Design review of the part built by this model. Coordinates are the model's own, in mm. Face numbers are marked on the shaded views. A direction names the side the tool comes from. Coordinates: 2 decimals unless noted, no trailing zeros. Write each loop counter-clockwise with the first axis right and the second up, starting at its lowest first coordinate (ties: lowest second). Pieces come first, ordered by that corner, then holes. Notation, with made-up numbers: M 41,36.5 L 89,36.5 A13 cw 89,53.5 Z; hole C 9,15.5 d10. An arc over 180 degrees is marked long. Write each question's results on one line, items separated by ' | '. Start each with the question number.
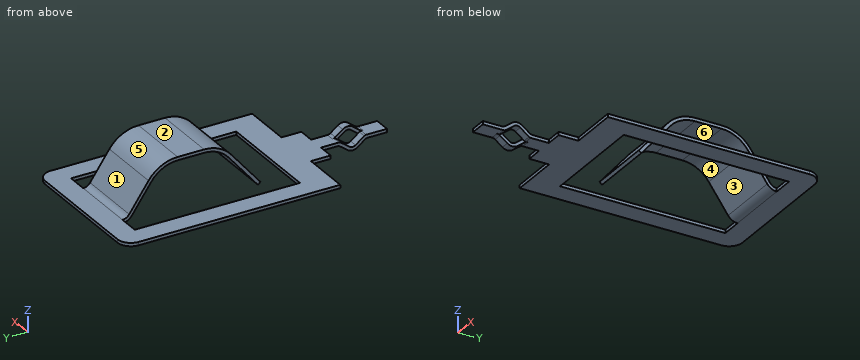
```python
from build123d import *

# Parameters (mm, degrees)
SKETCH1_W           = 6.5
SKETCH1_H           = 10
BOSS_EXTRUDE1_DEPTH = 0.2
BOSS_EXTRUDE2_DEPTH = 2
BOSS_EXTRUDE3_DEPTH = 0.5
FILLET1_R           = 0.8
BOSS_EXTRUDE7_DEPTH = 0.5


with BuildPart() as part:
    # Sketch1 → Boss-Extrude1 (new body)
    with BuildSketch(Plane.XY):
        Polygon((-4.5, 0), (4.5, 0), (4.5, -13), (1.5, -13), (1.5, -14.2), (-1.5, -14.2), (-1.5, -13), (-4.5, -13), align=None)
        with Locations((0, -6.3)):
            Rectangle(SKETCH1_W, SKETCH1_H, mode=Mode.SUBTRACT)
    extrude(amount=BOSS_EXTRUDE1_DEPTH)

    # Sketch2 → Boss-Extrude2 (add, symmetric)
    with BuildSketch(Plane.ZY):
        with BuildLine():
            Line((2.8, -4.64068371), (2.8, -6.24068371))
            ThreePointArc((2.8, -6.24068371), (2.617192211, -7.065276361), (2.103024175, -7.73535319))
            Line((2.103024175, -7.73535319), (0, -9.5))
            Line((0, -9.5), (0.128557522, -9.653208889))
            Line((0.128557522, -9.653208889), (2.231581697, -7.888562079))
            ThreePointArc((2.231581697, -7.888562079), (2.798453768, -7.149800013), (3, -6.24068371))
            Line((3, -6.24068371), (3, -4.64068371))
            ThreePointArc((3, -4.64068371), (2.756943079, -3.647392057), (2.082697913, -2.878562796))
            Line((2.082697913, -2.878562796), (0.413211782, -1.709576022))
            ThreePointArc((0.413211782, -1.709576022), (0.256494583, -1.530874307), (0.2, -1.3))
            Line((0.2, -1.3), (0, -1.3))
            ThreePointArc((0, -1.3), (0.079092417, -1.623224029), (0.298496495, -1.873406431))
            Line((0.298496495, -1.873406431), (1.967982626, -3.042393205))
            ThreePointArc((1.967982626, -3.042393205), (2.579540912, -3.73974178), (2.8, -4.64068371))
        make_face()
    extrude(amount=BOSS_EXTRUDE2_DEPTH, both=True)

    # Sketch4 → Boss-Extrude3 (add)
    with BuildSketch(Plane.ZY):
        with BuildLine():
            Line((0.2, -14.2), (0, -14.2))
            Line((0, -14.2), (0, -15.295761219))
            ThreePointArc((0, -15.295761219), (0.009055652, -15.351444505), (0.035289283, -15.401388772))
            Line((0.035289283, -15.401388772), (0.436234874, -15.93446579))
            ThreePointArc((0.436234874, -15.93446579), (0.496480735, -16.114793139), (0.436234874, -16.295120487))
            Line((0.436234874, -16.295120487), (0.035289283, -16.828197505))
            ThreePointArc((0.035289283, -16.828197505), (0.009055652, -16.878141772), (0, -16.933825058))
            Line((0, -16.933825058), (0, -18.2))
            Line((0, -18.2), (0.2, -18.2))
            Line((0.2, -18.2), (0.2, -17.042162177))
            ThreePointArc((0.2, -17.042162177), (0.215459808, -16.947099676), (0.260245861, -16.861834829))
            Line((0.260245861, -16.861834829), (0.596070967, -16.415338719))
            ThreePointArc((0.596070967, -16.415338719), (0.696480735, -16.114793139), (0.596070967, -15.814247558))
            Line((0.596070967, -15.814247558), (0.260245861, -15.367751448))
            ThreePointArc((0.260245861, -15.367751448), (0.215459808, -15.282486601), (0.2, -15.1874241))
            Line((0.2, -15.1874241), (0.2, -14.2))
        make_face()
    extrude(amount=-BOSS_EXTRUDE3_DEPTH)

    # Fillet1
    fillet1_edges = [part.edges().sort_by_distance(p)[0] for p in [
        (-4.5, 0, 0.1),
        (4.5, 0, 0.1),
    ]]
    fillet(fillet1_edges, radius=FILLET1_R)

    # Sketch7 → Boss-Extrude7 (add)
    with BuildSketch(Plane.ZY):
        with BuildLine():
            Line((0, -14.2), (0.2, -14.2))
            Line((0.2, -14.2), (0.2, -15.295761219))
            ThreePointArc((0.2, -15.295761219), (0.190944348, -15.351444505), (0.164710717, -15.401388772))
            Line((0.164710717, -15.401388772), (-0.236234874, -15.93446579))
            ThreePointArc((-0.236234874, -15.93446579), (-0.296480735, -16.114793139), (-0.236234874, -16.295120487))
            Line((-0.236234874, -16.295120487), (0.164710717, -16.828197505))
            ThreePointArc((0.164710717, -16.828197505), (0.190944348, -16.878141772), (0.2, -16.933825058))
            Line((0.2, -16.933825058), (0.2, -18.2))
            Line((0.2, -18.2), (0, -18.2))
            Line((0, -18.2), (0, -17.042162177))
            ThreePointArc((0, -17.042162177), (-0.015459808, -16.947099676), (-0.060245861, -16.861834829))
            Line((-0.060245861, -16.861834829), (-0.396070967, -16.415338719))
            ThreePointArc((-0.396070967, -16.415338719), (-0.496480735, -16.114793139), (-0.396070967, -15.814247558))
            Line((-0.396070967, -15.814247558), (-0.060245861, -15.367751448))
            ThreePointArc((-0.060245861, -15.367751448), (-0.015459808, -15.282486601), (0, -15.1874241))
            Line((0, -15.1874241), (0, -14.2))
        make_face()
    extrude(amount=BOSS_EXTRUDE7_DEPTH)


solid = part.part
```
Item 1: We need section A-A on x = -3. State the section outline as (y, z) points, then the cut area to 3 significant figures.
Item 2: We need section D-D on x = 3.5. State the section outline as (y, z) points, then the cut area to 3 significant figures.
Item 3: Draft analysis for pull direction Y (two halves, no side actions). For the marked faces 1, 2, 3 and 4, state which applies: released by +Y, released by -Y, zero draft, split by the parting line, or undercut.
Item 4: For the marked faces 5 and 6, list the 3-axis set-ups (+Z, -Z, +X, -X, +Y, -Y) from which the entire face can be reached by the end or side of a thin tool; tool diameter is ignored.
Item 5: We need section C-C on z = 1. State the section outline as (x, y) points, then the cut area to 3 significant figures.
Item 6: Insertion check: pin 1 Ø2 at (x, y) = (2, -9) entering from +Z; pin 2 Ø0.5 at (x, y) = (0, -18) entering from +Z; pin 3 Ø0.8 at (x, y) = (0, -18) entering from -Z. Each pin has a flat end and moves straight along its axis. Give the tip position at first contact, or say it passes through.
Item 7: Wall thickness on L1, parallel to Z at x = -3, y = -12.25; L2, parallel to Y at x = -0.5, z = 0.7; L3, parallel to Z at x = 1.5, y = -6: over which ranges is each line inside the solid? List them lowest first.
Item 8: We need section B-B on y = -4. State the section outline as (x, z) points.
Answer:
1) outline: M -13,0 L -11.3,0 L -11.3,0.2 L -13,0.2 Z; M -1.3,0 L 0,0 L 0,0.2 L -1.3,0.2 Z | area: 0.600 mm^2
2) outline: M -13,0 L 0,0 L 0,0.2 L -13,0.2 Z | area: 2.60 mm^2
3) face 1: released by +Y | face 2: zero draft | face 3: undercut | face 4: undercut
4) face 5: +Z, +X, -X, +Y | face 6: -Z, +X, -X
5) outline: M -2,-8.92 L 2,-8.92 L 2,-8.66 L -2,-8.66 Z; M -2,-2.36 L 2,-2.36 L 2,-2.12 L -2,-2.12 Z | area: 2.02 mm^2
6) pin 1: stops at z = 2.1 | pin 2: stops at z = 0.2 | pin 3: stops at z = 0
7) L1: z = 0 to 0.2 | L2: y = -9.17 to -8.91, -2.15 to -1.91 | L3: z = 2.8 to 3
8) outline: M -4.5,0 L -3.25,0 L -3.25,0.2 L -4.5,0.2 Z; M -2,2.69 L 2,2.69 L 2,2.9 L -2,2.9 Z; M 3.25,0 L 4.5,0 L 4.5,0.2 L 3.25,0.2 Z
